Here's how the part is built. I have some questions about the finished solid (model axes, mm). Face numbers are marked on the shaded views. A direction names the side the tool comes from. Coordinates: 2 decimals unless noted, no trailing zeros. Write each loop counter-clockwise with the first axis right and the second up, starting at its lowest first coordinate (ties: lowest second). Pieces come first, ordered by that corner, then holes.
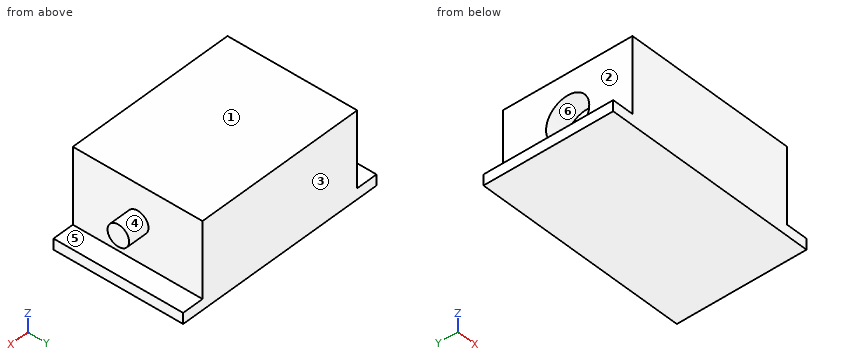
```python
from build123d import *

# Parameters (mm, degrees)
SKETCH1_W           = 100
SKETCH1_H           = 60
BOSS_EXTRUDE1_DEPTH = 40
SKETCH2_W           = 10
SKETCH2_H           = 35
CUT_EXTRUDE1_DEPTH  = 124.288280059
SKETCH3_R           = 10
CUT_EXTRUDE2_DEPTH  = 10
SKETCH4_R           = 5
BOSS_EXTRUDE2_DEPTH = 10


with BuildPart() as part:
    # Sketch1 → Boss-Extrude1 (new body)
    with BuildSketch(Plane.XY):
        with Locations((50, 30)):
            Rectangle(SKETCH1_W, SKETCH1_H)
    extrude(amount=BOSS_EXTRUDE1_DEPTH)

    # Sketch2 → Cut-Extrude1 (cut, through all)
    with BuildSketch(Plane.XZ):
        with Locations((5, 22.5)):
            Rectangle(SKETCH2_W, SKETCH2_H)
        with Locations((95, 22.5)):
            Rectangle(SKETCH2_W, SKETCH2_H)
    extrude(amount=-CUT_EXTRUDE1_DEPTH, mode=Mode.SUBTRACT)

    # Sketch3 → Cut-Extrude2 (cut)
    with BuildSketch(Plane.ZY.offset(-10)):
        with Locations((20, 30)):
            Circle(SKETCH3_R)
    extrude(amount=-CUT_EXTRUDE2_DEPTH, mode=Mode.SUBTRACT)

    # Sketch4 → Boss-Extrude2 (add)
    with BuildSketch(Plane(origin=(90, 0, 0), x_dir=(0, 0, -1), z_dir=(1, 0, 0))):
        with Locations(Location((-23, 30, 0), (0, 0, 180))):
            Circle(SKETCH4_R)
    extrude(amount=BOSS_EXTRUDE2_DEPTH)


solid = part.part
```
1) Imagine slicing it at C-C on z = 20. Please give me the cut outline in (x, y).
Values follow:
outline: (10, 0) - (90, 0) - (90, 26) - (100, 26) - (100, 34) - (90, 34) - (90, 60) - (10, 60) - (10, 40) - (20, 40) - (20, 20) - (10, 20) - close
2) I need wall thicknesses on probe 1 along Y at (x, z) = (16.5, 20); probe 2 along X at (y, z) = (27, 10); probe 3 along X at (y, z) = (27, 29). Which ranges of each line are inside material? Lowest first, please.
Values follow:
probe 1: y = 0 to 20, 40 to 60
probe 2: x = 10 to 90
probe 3: x = 20 to 90
3) We'd pull the mould along Y, two halves only. Please class the marked faces 3, 4, 5 and 6: pulls with the +Y half, pulls with the -Y half, needs draft (parallel to the pull), parting line crosses it, or undercut.
Values follow:
face 3: pulls with the +Y half
face 4: parting line crosses it
face 5: needs draft
face 6: undercut
4) Imagine slicing it at A-A on x = 91.5. Please give me the cut outline in (y, z), then the cut area to 3 significant figures.
Values follow:
outline: (0, 0) - (60, 0) - (60, 5) - (0, 5) - close; circle Ø10 at (30, 23)
area: 379 mm2
5) Will these pins go through, and if not, where does the flat tip stop? pin 1 (17.5 mm diameter, centred on y = 40, z = 21.5, fed in from -X); pin 2 (8 mm diameter, centred on x = 96.5, y = 38, fed in from +Z); pin 3 (5 mm diameter, centred on y = 50.5, z = 23.5, fed in from +X).
Values follow:
pin 1: stops at x = 10
pin 2: stops at z = 26
pin 3: stops at x = 90
6) Imagine slicing it at D-D on y = 36. Please give me the cut outline in (x, z).
Values follow:
outline: (0, 0) - (100, 0) - (100, 5) - (90, 5) - (90, 40) - (10, 40) - (10, 28) - (20, 28) - (20, 12) - (10, 12) - (10, 5) - (0, 5) - close
7) Imagine slicing it at B-B on y = 52. Please give me the cut outline in (x, z).
Values follow:
outline: (0, 0) - (100, 0) - (100, 5) - (90, 5) - (90, 40) - (10, 40) - (10, 5) - (0, 5) - close
8) On a 3-axis mill with a long thin cutter (end or side, diameter ignored), from which of +Z, -Z, +X, -X, +Y, -Y can I reach the whole of each face in a straight line? I mean the marked faces 1 and 2. Say none if no direction works.
Values follow:
face 1: +Z, +X, -X, +Y, -Y
face 2: +Z, -X, +Y, -Y
